Check sheet for the modelled part. Datum: model origin and axes. Units: mm. A direction names the side the tool comes from. Round coordinates to 2 decimals unless told otherwise and drop trailing zeros. Loops run counter-clockwise (first coordinate to the right, second up) from the corner with the lowest first, then second, coordinate; pieces in that order, holes last. Notation, with made-up numbers: (51.25, -27) -> (78.25, -27) arc R23 ccw to (78.25, 11) -> close; hole circle Ø2 at (5, 82). An arc over 180 degrees is marked (long way). Return JSON: item names as keys, results as strings.
from build123d import *

# Parameters (mm, degrees)
BOSS_EXTRUDE1_OUTLINE_R   = 2.5
BOSS_EXTRUDE1_OUTLINE_R_2 = 1.75
BOSS_EXTRUDE1_DEPTH       = 4.21
BOSS_EXTRUDE2_START       = 4.21
BOSS_EXTRUDE2_OUTLINE_R   = 2.5
BOSS_EXTRUDE2_OUTLINE_R_2 = 1.75
BOSS_EXTRUDE2_DEPTH       = 5.539999985
BOSS_EXTRUDE3_START       = -2.1
SKETCH3_W                 = 36.654989836
SKETCH3_H                 = 39.3126
SKETCH3_R                 = 2.5
SKETCH3_R_2               = 3.25
SKETCH3_W_2               = 9.43005
SKETCH3_H_2               = 9.2
SKETCH3_W_3               = 9.07015
SKETCH3_H_3               = 11.10254
BOSS_EXTRUDE3_DEPTH       = 2.1
CUT_EXTRUDE1_START        = -6
SKETCH3_2_R               = 3.25
SKETCH3_2_R_2             = 1.75
CUT_EXTRUDE1_DEPTH        = 6
SKETCH5_R                 = 4.3
CUT_EXTRUDE2_DEPTH        = 5
CHAMFER1_SIZE             = 3
CUT_EXTRUDE3_REACH        = 44.72
SKETCH6_W                 = 2.25
SKETCH6_H                 = 11.58
BOSS_EXTRUDE5_START       = 1.9
SKETCH7_W                 = 36.654989836
SKETCH7_H                 = 39.3126
SKETCH7_R                 = 4.3
SKETCH7_R_2               = 3.25
SKETCH7_W_2               = 10.43005
SKETCH7_H_2               = 10.2
SKETCH7_W_3               = 9.07015
SKETCH7_H_3               = 11.10254
SKETCH7_W_4               = 9.43005
SKETCH7_H_4               = 9.2
SKETCH7_R_3               = 4.225
BOSS_EXTRUDE5_DEPTH       = 1.9


# Read off the part's stored shape, not the designer's step: Boss-Extrude1, Boss-Extrude2
with BuildPart() as part:
    # Boss-Extrude1 outline → Boss-Extrude1 (new body)
    # profile 1 of 2: a face of its own
    with BuildSketch(Plane.XY):
        Polygon((17.1132, 10.4965), (17.1132, 5.1225), (18.7132, 5.1225), (18.7132, 19.6563), (-17.941789836, 19.6563), (-17.941789836, 4.917774053), (-17.1132, 4.917774053), (-17.1132, 10.4965), align=None)
        with Locations((-12.941789836, 14.6563)):
            Circle(BOSS_EXTRUDE1_OUTLINE_R, mode=Mode.SUBTRACT)
        with Locations((0.4826, 13.6525)):
            Circle(BOSS_EXTRUDE1_OUTLINE_R_2, mode=Mode.SUBTRACT)
        with Locations((13.7132, 14.6563)):
            Circle(BOSS_EXTRUDE1_OUTLINE_R, mode=Mode.SUBTRACT)
    # profile 2 of 2: a face of its own
    with BuildSketch(Plane.XY):
        Polygon((18.7132, -19.6563), (18.7132, -5.7575), (17.109037456, -5.7575), (17.105585288, -10.521897241), (-17.120805727, -10.497097621), (-17.116838767, -5.022225947), (-17.941789836, -5.022225947), (-17.941789836, -19.6563), align=None)
        with Locations((-12.941789836, -14.6563)):
            Circle(BOSS_EXTRUDE1_OUTLINE_R, mode=Mode.SUBTRACT)
        with Locations((0.508, -13.6525)):
            Circle(BOSS_EXTRUDE1_OUTLINE_R_2, mode=Mode.SUBTRACT)
        with Locations((13.7132, -14.6563)):
            Circle(BOSS_EXTRUDE1_OUTLINE_R, mode=Mode.SUBTRACT)
    extrude(amount=BOSS_EXTRUDE1_DEPTH)

    # Boss-Extrude2 outline → Boss-Extrude2 (add)
    with BuildSketch(Plane.XY.offset(BOSS_EXTRUDE2_START)):
        Polygon((17.1132, 10.4965), (17.1132, 5.1225), (18.7132, 5.1225), (18.7132, 19.6563), (-17.941789836, 19.6563), (-17.941789836, -19.6563), (18.7132, -19.6563), (18.7132, -5.7575), (17.109037456, -5.7575), (17.105585288, -10.521897241), (-17.120805727, -10.497097621), (-17.1132, -0.000300188), (-17.1132, 10.4965), align=None)
        with Locations((-12.941789836, -14.6563)):
            Circle(BOSS_EXTRUDE2_OUTLINE_R, mode=Mode.SUBTRACT)
        with Locations((0.508, -13.6525)):
            Circle(BOSS_EXTRUDE2_OUTLINE_R_2, mode=Mode.SUBTRACT)
        with Locations((13.7132, -14.6563)):
            Circle(BOSS_EXTRUDE2_OUTLINE_R, mode=Mode.SUBTRACT)
        with Locations((-12.941789836, 14.6563)):
            Circle(BOSS_EXTRUDE2_OUTLINE_R, mode=Mode.SUBTRACT)
        with Locations((0.4826, 13.6525)):
            Circle(BOSS_EXTRUDE2_OUTLINE_R_2, mode=Mode.SUBTRACT)
        with Locations((13.7132, 14.6563)):
            Circle(BOSS_EXTRUDE2_OUTLINE_R, mode=Mode.SUBTRACT)
    extrude(amount=BOSS_EXTRUDE2_DEPTH)

    # Sketch3 → Boss-Extrude3 (add)
    with BuildSketch(Plane.XY.offset(9.749999985).offset(BOSS_EXTRUDE3_START)):
        with Locations((0.385705082, 0)):
            Rectangle(SKETCH3_W, SKETCH3_H)
        with Locations((-12.941789836, 14.6563)):
            Circle(SKETCH3_R, mode=Mode.SUBTRACT)
        with Locations((13.7132, 14.6563)):
            Circle(SKETCH3_R, mode=Mode.SUBTRACT)
        with Locations((-12.941789836, -14.6563)):
            Circle(SKETCH3_R, mode=Mode.SUBTRACT)
        with Locations((13.7132, -14.6563)):
            Circle(SKETCH3_R, mode=Mode.SUBTRACT)
        with Locations((0.508, -13.6525)):
            Circle(SKETCH3_R_2, mode=Mode.SUBTRACT)
        with Locations((0.4826, 13.6525)):
            Circle(SKETCH3_R_2, mode=Mode.SUBTRACT)
        with Locations((-12.398175, -0.6835)):
            Rectangle(SKETCH3_W_2, SKETCH3_H_2, mode=Mode.SUBTRACT)
        with Locations((12.357075, -0.28623)):
            Rectangle(SKETCH3_W_3, SKETCH3_H_3, mode=Mode.SUBTRACT)
    extrude(amount=BOSS_EXTRUDE3_DEPTH)

    # Sketch3<2> → Cut-Extrude1 (cut)
    # profile 1 of 2: a face of its own
    with BuildSketch(Plane.XY.offset(9.749999985).offset(CUT_EXTRUDE1_START)):
        with Locations((0.4826, 13.6525)):
            Circle(SKETCH3_2_R)
        with Locations((0.4826, 13.6525)):
            Circle(SKETCH3_2_R_2, mode=Mode.SUBTRACT)
    # profile 2 of 2: a face of its own
    with BuildSketch(Plane.XY.offset(9.749999985).offset(CUT_EXTRUDE1_START)):
        with Locations((0.508, -13.6525)):
            Circle(SKETCH3_2_R)
        with Locations((0.508, -13.6525)):
            Circle(SKETCH3_2_R_2, mode=Mode.SUBTRACT)
    extrude(amount=CUT_EXTRUDE1_DEPTH, mode=Mode.SUBTRACT)

    # Sketch5 → Cut-Extrude2 (cut)
    with BuildSketch(Plane.XY.offset(9.749999985)):
        with Locations((-12.941789836, 14.6563)):
            Circle(SKETCH5_R)
        with Locations((13.7132, 14.6563)):
            Circle(SKETCH5_R)
        with Locations((-12.941789836, -14.6563)):
            Circle(SKETCH5_R)
        with Locations((13.7132, -14.6563)):
            Circle(SKETCH5_R)
    extrude(amount=-CUT_EXTRUDE2_DEPTH, mode=Mode.SUBTRACT)

    # Chamfer1
    # the kernel refuses this chamfer: 3 mm, written as the material it takes off along each edge
    with BuildSketch(Plane(origin=(13.7132, 14.6563, 4.749999985), x_dir=(1, 0, 0), z_dir=(0, 1, 0))) as chamfer1_piece_1_section:
        Polygon((2.5 + CHAMFER1_SIZE, 0), (2.5, CHAMFER1_SIZE), (2.5, 0), align=None)
    chamfer1_piece_1 = revolve(axis=Axis((13.7132, 14.6563, 4.749999985), (0, 0, -1)), mode=Mode.PRIVATE)
    chamfer1_piece_1 = chamfer1_piece_1 & Plane(origin=(13.7132, 14.6563, 2.638456685), x_dir=(1, 0, 0), z_dir=(0, 0, 1)) * Cylinder(4.3, 22, mode=Mode.PRIVATE)
    add(chamfer1_piece_1, mode=Mode.SUBTRACT)
    with BuildSketch(Plane(origin=(-12.941789836, -14.6563, 4.749999985), x_dir=(1, 0, 0), z_dir=(0, 1, 0))) as chamfer1_piece_2_section:
        Polygon((2.5 + CHAMFER1_SIZE, 0), (2.5, CHAMFER1_SIZE), (2.5, 0), align=None)
    chamfer1_piece_2 = revolve(axis=Axis((-12.941789836, -14.6563, 4.749999985), (0, 0, -1)), mode=Mode.PRIVATE)
    chamfer1_piece_2 = chamfer1_piece_2 & Plane(origin=(-12.941789836, -14.6563, 2.638456685), x_dir=(1, 0, 0), z_dir=(0, 0, 1)) * Cylinder(4.3, 22, mode=Mode.PRIVATE)
    add(chamfer1_piece_2, mode=Mode.SUBTRACT)
    with BuildSketch(Plane(origin=(13.7132, -14.6563, 4.749999985), x_dir=(1, 0, 0), z_dir=(0, 1, 0))) as chamfer1_piece_3_section:
        Polygon((2.5 + CHAMFER1_SIZE, 0), (2.5, CHAMFER1_SIZE), (2.5, 0), align=None)
    chamfer1_piece_3 = revolve(axis=Axis((13.7132, -14.6563, 4.749999985), (0, 0, -1)), mode=Mode.PRIVATE)
    chamfer1_piece_3 = chamfer1_piece_3 & Plane(origin=(13.7132, -14.6563, 2.638456685), x_dir=(1, 0, 0), z_dir=(0, 0, 1)) * Cylinder(4.3, 22, mode=Mode.PRIVATE)
    add(chamfer1_piece_3, mode=Mode.SUBTRACT)
    with BuildSketch(Plane(origin=(-12.941789836, 14.6563, 4.749999985), x_dir=(1, 0, 0), z_dir=(0, 1, 0))) as chamfer1_piece_4_section:
        Polygon((2.5 + CHAMFER1_SIZE, 0), (2.5, CHAMFER1_SIZE), (2.5, 0), align=None)
    chamfer1_piece_4 = revolve(axis=Axis((-12.941789836, 14.6563, 4.749999985), (0, 0, -1)), mode=Mode.PRIVATE)
    chamfer1_piece_4 = chamfer1_piece_4 & Plane(origin=(-12.941789836, 14.6563, 2.638456685), x_dir=(1, 0, 0), z_dir=(0, 0, 1)) * Cylinder(4.3, 22, mode=Mode.PRIVATE)
    add(chamfer1_piece_4, mode=Mode.SUBTRACT)

    # Cut-Extrude3: up to this face of the body (flat: up to its plane)
    cut_extrude3_end = Plane(part.part.faces().sort_by_distance((-17.118822247, -7.759661784, 2.105))[0])
    # Sketch6 → Cut-Extrude3 (cut, up to the picked face)
    with BuildSketch(Plane.ZY.offset(17.941789836), mode=Mode.PRIVATE) as cut_extrude3_sk1:
        with Locations((7.124999985, -0.86020819)):
            Rectangle(SKETCH6_W, SKETCH6_H)
    cut_extrude3_tool1 = split(extrude(cut_extrude3_sk1.sketch, amount=-CUT_EXTRUDE3_REACH, mode=Mode.PRIVATE), bisect_by=cut_extrude3_end, keep=Keep.BOTH, mode=Mode.PRIVATE)
    add(cut_extrude3_tool1.solids().sort_by(Axis((-17.94179, -0.860208, 7.125), (1, 0, 0)))[0], mode=Mode.SUBTRACT)

    # Sketch7 → Boss-Extrude5 (add)
    # profile 1 of 3: a face of its own
    with BuildSketch(Plane.XY.offset(9.749999985).offset(BOSS_EXTRUDE5_START)):
        with Locations((0.385705082, 0)):
            Rectangle(SKETCH7_W, SKETCH7_H)
        with Locations((13.7132, 14.6563)):
            Circle(SKETCH7_R, mode=Mode.SUBTRACT)
        with Locations((13.7132, -14.6563)):
            Circle(SKETCH7_R, mode=Mode.SUBTRACT)
        with Locations((0.4826, 13.6525)):
            Circle(SKETCH7_R_2, mode=Mode.SUBTRACT)
        with Locations((0.508, -13.6525)):
            Circle(SKETCH7_R_2, mode=Mode.SUBTRACT)
        with Locations((-12.941789836, 14.6563)):
            Circle(SKETCH7_R, mode=Mode.SUBTRACT)
        with Locations((-12.941789836, -14.6563)):
            Circle(SKETCH7_R, mode=Mode.SUBTRACT)
        with Locations((-12.398175, -0.6835)):
            Rectangle(SKETCH7_W_2, SKETCH7_H_2, mode=Mode.SUBTRACT)
        with Locations((12.357075, -0.28623)):
            Rectangle(SKETCH7_W_3, SKETCH7_H_3, mode=Mode.SUBTRACT)
    # profile 2 of 3: a face of its own
    with BuildSketch(Plane.XY.offset(9.749999985).offset(BOSS_EXTRUDE5_START)):
        with Locations((-12.398175, -0.6835)):
            Rectangle(SKETCH7_W_2, SKETCH7_H_2)
        with Locations((-12.398175, -0.6835)):
            Rectangle(SKETCH7_W_4, SKETCH7_H_4, mode=Mode.SUBTRACT)
    # profile 3 of 3: a face of its own
    with BuildSketch(Plane.XY.offset(9.749999985).offset(BOSS_EXTRUDE5_START)):
        with Locations((-12.398175, -0.6835)):
            Rectangle(SKETCH7_W_4, SKETCH7_H_4)
        with Locations((-12.88315, -0.6835)):
            Circle(SKETCH7_R_3, mode=Mode.SUBTRACT)
    extrude(amount=-BOSS_EXTRUDE5_DEPTH)


solid = part.part
Q1. Draft check along X on faces 1 (the flat face through (0, -17, 0)), 2 (the flat face through (2, -15, 3.75)), 3 (the flat face through (-12, 3.916, 9)). Enter one of: released by +X, released by -X, zero draft, split by the parting line, or undercut.
Results list:
{"face 1": "zero draft", "face 2": "undercut", "face 3": "undercut"}
Q2. Material ranges on line 1 (X direction, y = -5, z = 8.5); line 2 (Y direction, x = -0.5, z = 1.25); line 3 (X direction, y = 6, z = 5.25), recorded low to high.
Results list:
{"line 1": "-17.94 to -17.11, -7.68 to 7.82, 16.89 to 18.71", "line 2": "-19.66 to -15.08, -12.22 to -10.51, 10.5 to 12.2, 15.1 to 19.66", "line 3": "-17.94 to -17.11, 17.11 to 18.71"}
Q3. Tool access check on faces 4 (the flat face through (2, 12, 3.75)), 5 (the flat face through (-17.5, 4.918, 2.1)), 6 (the flat face through (-7.683, -1, 9)). Record the directions out of +Z, -Z, +X, -X, +Y, -Y that give a thin tool (end or side, any length) a straight path to the whole face; none if there is none.
Results list:
{"face 4": "+Z", "face 5": "-Z, +X, -X", "face 6": "-Z"}
Q4. Section check B-B (z = 9). Count the separate pieces of the cut face and the enclosed holes in it, then the cut area to 3 significant figures.
Results list:
{"separate pieces": "1", "enclosed holes": "8", "area": "955 mm^2"}
Q5. Section check A-A (z = 1). Record the boundary of the cut face in (x, y).
Results list:
{"outline": "(-17.94, -19.66) -> (18.71, -19.66) -> (18.71, -5.76) -> (17.11, -5.76) -> (17.11, -10.52) -> (-17.12, -10.5) -> (-17.12, -5.02) -> (-17.94, -5.02) -> close; (-17.94, 4.92) -> (-17.11, 4.92) -> (-17.11, 10.5) -> (17.11, 10.5) -> (17.11, 5.12) -> (18.71, 5.12) -> (18.71, 19.66) -> (-17.94, 19.66) -> close; hole circle Ø5 at (-12.94, -14.66); hole circle Ø5 at (-12.94, 14.66); hole circle Ø3.5 at (0.48, 13.65); hole circle Ø3.5 at (0.51, -13.65); hole circle Ø5 at (13.71, -14.66); hole circle Ø5 at (13.71, 14.66)"}
Q6. Go/stop test with flat-tipped pins: pin 1 (3 mm diameter, centred on x = 0.51, y = -13.65, fed in from -Z); pin 2 (8 mm diameter, centred on x = -12.94, y = -14.66, fed in from +Z). Record where each tip stops, or that it passes through.
Results list:
{"pin 1": "through", "pin 2": "z = 3.25"}
